from build123d import *

# Parameters (mm, degrees)
SKETCH2_W               = 230
SKETCH2_H               = 148
BOSS_EXTRUDE1_DEPTH     = 40
CUT_EXTRUDE2_DEPTH      = 126
SHELL2_T                = -3
SKETCH6_R               = 16
SKETCH6_R_2             = 6
SKETCH6_R_3             = 2
SKETCH6_R_4             = 6.65813103
SKETCH6_R_5             = 2.01097319
CUT_EXTRUDE3_DEPTH      = 126
SKETCH8_W               = 15
SKETCH8_H               = 47.399828673
CUT_EXTRUDE4_DEPTH      = 10
SKETCH12_R              = 8.5
CUT_EXTRUDE7_DEPTH      = 4
CUT_EXTRUDE7_DEPTH_BACK = 13
SKETCH13_R              = 8.5
CUT_EXTRUDE8_DEPTH      = 10
SKETCH14_R              = 8.5
CUT_EXTRUDE9_DEPTH      = 10
SKETCH15_R              = 8.5
CUT_EXTRUDE10_DEPTH     = 10
SKETCH16_R              = 8.5
CUT_EXTRUDE11_DEPTH     = 10
SKETCH17_R              = 8.5
CUT_EXTRUDE12_DEPTH     = 10
SKETCH18_R              = 8.5
CUT_EXTRUDE13_DEPTH     = 10
SKETCH19_R              = 8.5
CUT_EXTRUDE14_DEPTH     = 10
SKETCH23_W              = 37.252555384
SKETCH23_H              = 4.191255607
BOSS_EXTRUDE2_DEPTH     = 15
BOSS_EXTRUDE3_DEPTH     = 37.252555


with BuildPart() as part:
    # Sketch2 → Boss-Extrude1 (new body)
    with BuildSketch(Plane(origin=(0, 0, 0), x_dir=(1, 0, 0), z_dir=(0, 1, 0))):
        Rectangle(SKETCH2_W, SKETCH2_H)
    extrude(amount=BOSS_EXTRUDE1_DEPTH)

    # Sketch4 → Cut-Extrude2 (cut)
    with BuildSketch(Plane(origin=(0, 40, 0), x_dir=(1, 0, 0), z_dir=(0, 1, 0))):
        Polygon((-79.644660941, 74), (-115, 38.644660941), (-115, 74), align=None)
        Polygon((115, 74), (79.644660941, 74), (115, 38.644660941), align=None)
        Polygon((115, -38.644660941), (115, -74), (79.644660941, -74), align=None)
        Polygon((-115, -74), (-79.644660941, -74), (-115, -38.644660941), align=None)
    extrude(amount=-CUT_EXTRUDE2_DEPTH, mode=Mode.SUBTRACT)

    # Shell2
    shell2_openings = [part.faces().sort_by_distance(p)[0] for p in [
        (0, 40, 0),
    ]]
    offset(amount=SHELL2_T, openings=shell2_openings, kind=Kind.INTERSECTION)

    # Sketch6 → Cut-Extrude3 (cut)
    with BuildSketch(Plane.XZ):
        with Locations((24.697986577, 0)):
            Circle(SKETCH6_R)
        with Locations((8.697986577, 25.5)):
            Circle(SKETCH6_R_2)
        with Locations((45, 27.5)):
            Circle(SKETCH6_R_3)
        with Locations((8.697986577, -25.5)):
            Circle(SKETCH6_R_4)
        with Locations((45, -27.5)):
            Circle(SKETCH6_R_5)
    extrude(amount=-CUT_EXTRUDE3_DEPTH, mode=Mode.SUBTRACT)

    # Sketch8 → Cut-Extrude4 (cut)
    with BuildSketch(Plane(origin=(0, 3, 0), x_dir=(1, 0, 0), z_dir=(0, 1, 0))):
        Polygon((-75.93928893, 71), (-29.973726036, 71), (-29.973726036, 56), (-72.188816818, 56), (-101.393398282, 26.795418536), (-112, 37.402020254), (-78.402020254, 71), align=None)
        with Locations((104.5, -0.132528068)):
            Rectangle(SKETCH8_W, SKETCH8_H)
        with Locations((-104.5, -0.132528068)):
            Rectangle(SKETCH8_W, SKETCH8_H)
        Polygon((101.393398282, 26.795418536), (72.188816818, 56), (29.973726036, 56), (29.973726036, 71), (75.93928893, 71), (78.402020254, 71), (112, 37.402020254), align=None)
        Polygon((112, -37.402020254), (101.393398282, -26.795418536), (72.188816818, -56), (29.973726036, -56), (29.973726036, -71), (75.93928893, -71), (78.402020254, -71), align=None)
        Polygon((-101.393398282, -26.795418536), (-72.188816818, -56), (-29.973726036, -56), (-29.973726036, -71), (-75.93928893, -71), (-78.402020254, -71), (-112, -37.402020254), align=None)
    extrude(amount=-CUT_EXTRUDE4_DEPTH, mode=Mode.SUBTRACT)

    # Sketch12 → Cut-Extrude7 (cut, two sides)
    with BuildSketch(Plane.XY.offset(74)) as cut_extrude7_sk:
        with Locations((-65.902020254, 10)):
            Circle(SKETCH12_R)
        with Locations((-39.902020254, 10)):
            Circle(SKETCH12_R)
        with Locations((39.902020254, 10)):
            Circle(SKETCH12_R)
        with Locations((65.902020254, 10)):
            Circle(SKETCH12_R)
    extrude(amount=CUT_EXTRUDE7_DEPTH, mode=Mode.SUBTRACT)
    extrude(cut_extrude7_sk.sketch, amount=-CUT_EXTRUDE7_DEPTH_BACK, mode=Mode.SUBTRACT)

    # Sketch13 → Cut-Extrude8 (cut)
    with BuildSketch(Plane(origin=(0, 0, -74), x_dir=(-1, 0, 0), z_dir=(0, 0, -1))):
        with Locations((-39.902020254, 10)):
            Circle(SKETCH13_R)
        with Locations((-65.902020254, 10)):
            Circle(SKETCH13_R)
        with Locations((39.902020254, 10)):
            Circle(SKETCH13_R)
        with Locations((65.902020254, 10)):
            Circle(SKETCH13_R)
    extrude(amount=-CUT_EXTRUDE8_DEPTH, mode=Mode.SUBTRACT)

    # Sketch14 → Cut-Extrude9 (cut)
    with BuildSketch(Plane.ZY.offset(115)):
        with Locations((12.997979746, 10)):
            Circle(SKETCH14_R)
        with Locations((-13.002020254, 10)):
            Circle(SKETCH14_R)
    extrude(amount=-CUT_EXTRUDE9_DEPTH, mode=Mode.SUBTRACT)

    # Sketch15 → Cut-Extrude10 (cut)
    with BuildSketch(Plane(origin=(-76.82233047, 0, -76.82233047), x_dir=(-0.707106781, 0, 0.707106781), z_dir=(-0.707106781, 0, -0.707106781))):
        with Locations((14.734018716, 10)):
            Circle(SKETCH15_R)
        with Locations((40.734018716, 10)):
            Circle(SKETCH15_R)
    extrude(amount=-CUT_EXTRUDE10_DEPTH, mode=Mode.SUBTRACT)

    # Sketch16 → Cut-Extrude11 (cut)
    with BuildSketch(Plane(origin=(-76.82233047, 0, 76.82233047), x_dir=(0.707106781, 0, 0.707106781), z_dir=(-0.707106781, 0, 0.707106781))):
        with Locations((-40.734018716, 10)):
            Circle(SKETCH16_R)
        with Locations((-14.734018716, 10)):
            Circle(SKETCH16_R)
    extrude(amount=-CUT_EXTRUDE11_DEPTH, mode=Mode.SUBTRACT)

    # Sketch17 → Cut-Extrude12 (cut)
    with BuildSketch(Plane(origin=(115, 0, 0), x_dir=(0, 0, -1), z_dir=(1, 0, 0))):
        with Locations((13.002020254, 10)):
            Circle(SKETCH17_R)
        with Locations((-12.997979746, 10)):
            Circle(SKETCH17_R)
    extrude(amount=-CUT_EXTRUDE12_DEPTH, mode=Mode.SUBTRACT)

    # Sketch18 → Cut-Extrude13 (cut)
    with BuildSketch(Plane(origin=(76.82233047, 0, 76.82233047), x_dir=(0.707106781, 0, -0.707106781), z_dir=(0.707106781, 0, 0.707106781))):
        with Locations((40.734018716, 10)):
            Circle(SKETCH18_R)
        with Locations((14.734018716, 10)):
            Circle(SKETCH18_R)
    extrude(amount=-CUT_EXTRUDE13_DEPTH, mode=Mode.SUBTRACT)

    # Sketch19 → Cut-Extrude14 (cut)
    with BuildSketch(Plane(origin=(76.82233047, 0, -76.82233047), x_dir=(-0.707106781, 0, -0.707106781), z_dir=(0.707106781, 0, -0.707106781))):
        with Locations((-40.734018716, 10)):
            Circle(SKETCH19_R)
        with Locations((-14.734018716, 10)):
            Circle(SKETCH19_R)
    extrude(amount=-CUT_EXTRUDE14_DEPTH, mode=Mode.SUBTRACT)

    # Sketch23 → Boss-Extrude2 (add)
    with BuildSketch(Plane(origin=(-112, 0, 0), x_dir=(0, 0, -1), z_dir=(1, 0, 0))):
        with Locations((0, 37.904372197)):
            Rectangle(SKETCH23_W, SKETCH23_H)
    extrude(amount=BOSS_EXTRUDE2_DEPTH)

    # Sketch26 → Boss-Extrude3 (add)
    with BuildSketch(Plane.XY.offset(18.626277692)):
        Polygon((-112.232432426, 35.808744393), (-112.232432426, 22.816581324), (-97, 35.808744393), align=None)
    extrude(amount=-BOSS_EXTRUDE3_DEPTH)


solid = part.part
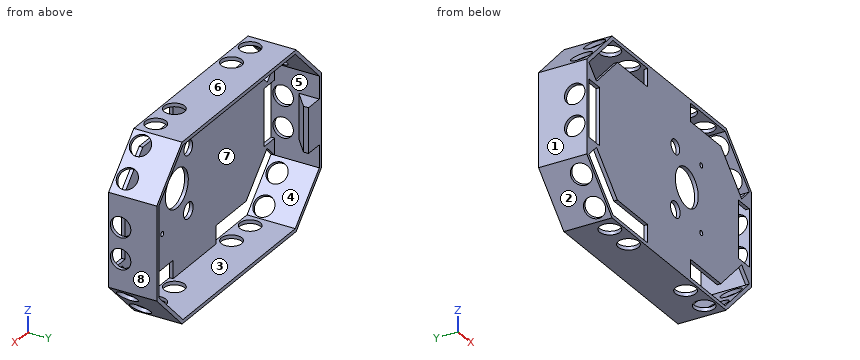
Build history of the part. All positions in model axes, mm. Face numbers are marked on the shaded views. A direction names the side the tool comes from. Coordinates: 2 decimals unless noted, no trailing zeros. Order: outer loops, then holes, each group sorted by start corner. A loop starts at its lowest first (then second) coordinate and runs counter-clockwise, first axis right, second up. Notation, with made-up numbers: (48, 36) - (65, 36) arc R16 cw to (65, 56) - close; hole circle Ø11 at (33, 2.25). An arc over 180 degrees is marked (long way). Write item = value, one per line. Start each with the question number.
1) 3-axis set-ups, long thin cutter, end or side, ignore diameter. For the marked faces 1, 2, 3, 4 and 5: which of +Z, -Z, +X, -X, +Y, -Y reach the whole face in a straight line?
2) Two-plate mould, pull along X, no slides. Class the marked faces 6, 7 and 8: pulls with the +X half, pulls with the -X half, needs draft (parallel to the pull), parting line crosses it, or undercut.
3) Saw through at A-A on z = 0. Write the cut outline in (x, y), then the cut area to 3 significant figures.
4) Saw through at D-D on z = -34.5. Write the cut outline in (x, y).
5) Flat gauge pins, fed straight in: pin 1 Ø10 at (x, z) = (-8, 57) entering from -Y; pin 2 Ø12 at (x, z) = (10.5, -37.5) entering from +Y; pin 3 Ø1 at (y, z) = (11.5, 7) entering from +X; pin 4 Ø3 at (y, z) = (14, -52.5) entering from -X. Where does each tip first touch, or does it go through?
6) Saw through at C-C on y = 28. Write the cut outline in (x, z).
7) Wall check: line 1 along Z through (x, y) = (45, 1.6); line 2 along X through (y, z) = (33.5, 31.5); line 3 along Z through (x, y) = (4, 13.5). Give the ranges that are in metal, low to high. Write a range as from..to.
8) Saw through at B-B on x = 37. Write the cut outline in (y, z), then the cut area to 3 significant figures.
From the geometry:
q1.face_1 = +Z, -Z, -X, +Y, -Y
q1.face_2 = -Z, -X, +Y, -Y
q1.face_3 = +Y
q1.face_4 = +Y, -Y
q1.face_5 = none
q2.face_6 = needs draft
q2.face_7 = undercut
q2.face_8 = pulls with the +X half
q3.outline = (-115, 0) - (-112, 0) - (-112, 23.01) - (-97, 35.81) - (-97, 40) - (-115, 40) - close; (-97, 0) - (8.7, 0) - (8.7, 3) - (-97, 3) - close; (40.7, 0) - (97, 0) - (97, 3) - (40.7, 3) - close; (112, 0) - (115, 0) - (115, 40) - (112, 40) - close
q3.area = 885 mm^2
q4.outline = (-115, 0) - (-109.1, 0) - (-109.1, 3) - (-112, 3) - (-112, 40) - (-115, 40) - close; (-93.69, 0) - (93.69, 0) - (93.69, 3) - (-93.69, 3) - close; (109.1, 0) - (115, 0) - (115, 40) - (112, 40) - (112, 3) - (109.1, 3) - close
q5.pin_1 = 0
q5.pin_2 = 3
q5.pin_3 = through
q5.pin_4 = -101.04
q6.outline = (-115, -38.64) - (-79.64, -74) - (79.64, -74) - (115, -38.64) - (115, 38.64) - (79.64, 74) - (-79.64, 74) - (-115, 38.64) - close; hole (-112, -37.4) - (-78.4, -71) - (78.4, -71) - (112, -37.4) - (112, 37.4) - (78.4, 71) - (-78.4, 71) - (-112, 37.4) - (-112, 18.63) - (-106.16, 18.63) - (-106.16, -18.63) - (-112, -18.63) - close
q7.line_1 = -74..-71, -56..-29.51, -25.49..25.5, 29.5..56, 71..74
q7.line_2 = -115..-112, 112..115
q7.line_3 = -74..-71, 71..74
q8.outline = (0, -74) - (2.01, -74) - (2.01, -71) - (0, -71) - close; (0, -56) - (3, -56) - (3, -10.23) - (0, -10.23) - close; (0, 10.23) - (3, 10.23) - (3, 56) - (0, 56) - close; (0, 71) - (2.01, 71) - (2.01, 74) - (0, 74) - close; (17.99, -74) - (40, -74) - (40, -71) - (17.99, -71) - close; (17.99, 71) - (40, 71) - (40, 74) - (17.99, 74) - close
q8.area = 419 mm^2
